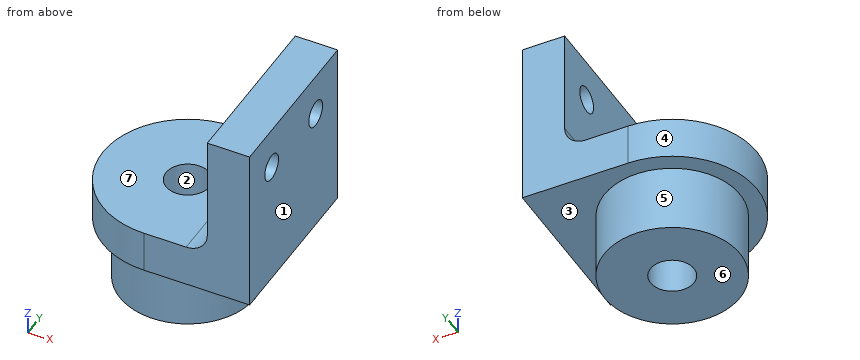
Autodesk Inventor part; units mm, degrees
ref_plane "YZ Plane" through (0, 0, 0) normal (1, 0, 0) x (0, 1, 0)
ref_plane "XZ Plane" through (0, 0, 0) normal (0, 1, 0) x (-1, 0, 0)
ref_plane "XY Plane" through (0, 0, 0) normal (0, 0, 1) x (1, 0, 0)
sketch "Sketch1" plane through (0, 0, 0) normal (0, 0, 1) x (1, 0, 0)
  circle A0 centre (0, 0) radius 10.16
  circle A1 centre (0, 0) radius 8.7376
  dimension "d0" = 20.32
  dimension "d6" = 17.4752
extrude "Extrusion1" add sketch "Sketch1" along normal blind 10.16 contours A0 | A1
sketch "Sketch2" plane through (0, 0, 10.16) normal (0, 0, 1) x (1, 0, 0)
  circle A0 centre (0, 0) radius 10.16
  circle A1 centre (0, 0) radius 12.7 construction
  line L0 (0, 12.7) -> (15.875, 12.7)
  line L1 (15.875, 12.7) -> (15.875, -12.7)
  line L2 (15.875, -12.7) -> (0, -12.7)
  arc A2 (0, 12.7) -> (0, -12.7) centre (0, 0) ccw
  point P0 (15.875, 0)
  dimension "d3" = 2.54
  dimension "d14" = 15.875
  dimension "d35" = 25.4
extrude "Extrusion2" add sketch "Sketch2" along normal blind 6.35 contours A0 | L0 L1 L2 A2
sketch "Sketch4" plane through (0, 0, 16.51) normal (0, 0, 1) x (1, 0, 0)
  arc A0 (0, 12.7) -> (0, -12.7) centre (0, 0) ccw
hole "Hole2" at (0, 0, 16.51) direction (0, 0, -1) diameter 6.5278 end through all
sketch "Sketch5" plane through (0, 0, 16.51) normal (0, 0, 1) x (1, 0, 0)
  line L0 (15.875, 12.7) -> (0, 12.7)
  line L1 (0, -12.7) -> (15.875, -12.7)
  line L2 (15.875, 12.7) -> (9.525, 12.7)
  line L3 (9.525, 12.7) -> (9.525, -12.7)
  line L4 (9.525, -12.7) -> (15.875, -12.7)
  line L5 (15.875, -12.7) -> (15.875, 12.7)
  point P0 (0, 0)
  dimension "d22" = 6.35
extrude "Extrusion3" add sketch "Sketch5" along normal blind 19.05
fillet "Fillet1" radius 3.175 1 edges at (9.525, 0, 16.51)
sketch "Sketch6" plane through (15.875, -12.7, 10.16) normal (1, 0, 0) x (0, 0, -1)
  line L0 (-19.05, 19.05) -> (-19.05, 6.35) construction
  line L1 (-25.4, 0) -> (-25.4, 25.4) construction
  line L2 (0, 25.4) -> (-25.4, 25.4) construction
  point P0 (10.16, 12.7)
  point P1 (-19.05, 12.7)
  point P2 (-25.4, 12.7)
  point P3 (-12.7, 25.4)
  dimension "d26" = 12.7
  dimension "d34" = 6.35
hole "Hole3" at (15.875, 6.35, 29.21) at (15.875, -6.35, 29.21) direction (-1, 0, 0) diameter 3.9624 end through all
properties part number "constant force Spring Holder" material "ABS Plastic"
Check sheet for the modelled part. Datum: model origin and axes. Units: mm. Face numbers are marked on the shaded views. A direction names the side the tool comes from. Round coordinates to 2 decimals unless told otherwise and drop trailing zeros. Loops run counter-clockwise (first coordinate to the right, second up) from the corner with the lowest first, then second, coordinate; pieces in that order, holes last.
1. Set-up check for the marked faces 5, 6 and 7: record each of +Z, -Z, +X, -X, +Y, -Y from which the full face is reachable in a straight line by a thin tool's end or side.
2. Gauge pin test, flat ends, axial feed: pin 1 Ø4.5 at (y, z) = (6.35, 29.21) entering from -X (3 decimals); pin 2 Ø3 at (x, y) = (-2.5, -0.5) entering from +Z; pin 3 Ø3 at (x, z) = (-4.5, 13.5) entering from +Y. Record the tip position at first contact, or that the pin passes through.
3. Sectioned sample at C-C on x = -2.5. Record the boundary of the cut face in (y, z).
4. Sectioned sample at B-B on y = 0. Record the boundary of the cut face in (x, z) (3 decimals).
5. Mould release check, pull along X, two halves, no side actions. Record for the marked faces 1, 2, 3 and 4: released by +X, released by -X, zero draft, split by the parting line, or undercut.
6. Sectioned sample at D-D on x = 4.25. Record the boundary of the cut face in (y, z).
7. Sectioned sample at A-A on z = 29.21. Record the boundary of the cut face in (x, y) (3 decimals), and give its area (3 significant figures).
8. Scan lines: probe 1 along Y at (x, z) = (14.75, 29.21); probe 2 along Y at (x, z) = (0, 5); probe 3 along Z at (x, y) = (14.25, -6.35). Record each from-to range of solid material in increasing order.
Recorded:
1. face 5: -Z
1. face 6: -Z, +X, -X, +Y, -Y
1. face 7: +Z, -X, +Y, -Y
2. pin 1: stops at x = 9.525
2. pin 2: stops at z = 16.51
2. pin 3: stops at y = 12.34
3. outline: (-12.45, 10.16) - (-9.85, 10.16) - (-9.85, 0) - (-2.1, 0) - (-2.1, 16.51) - (-12.45, 16.51) - close; (2.1, 0) - (9.85, 0) - (9.85, 10.16) - (12.45, 10.16) - (12.45, 16.51) - (2.1, 16.51) - close
4. outline: (-12.7, 10.16) - (-10.16, 10.16) - (-10.16, 0) - (-3.264, 0) - (-3.264, 16.51) - (-12.7, 16.51) - close; (3.264, 0) - (10.16, 0) - (10.16, 10.16) - (15.875, 10.16) - (15.875, 35.56) - (9.525, 35.56) - (9.525, 19.685) arc R3.175 cw to (6.35, 16.51) - (3.264, 16.51) - close
5. face 1: released by +X
5. face 2: undercut
5. face 3: zero draft
5. face 4: released by -X
6. outline: (-12.7, 10.16) - (-9.23, 10.16) - (-9.23, 0) - (9.23, 0) - (9.23, 10.16) - (12.7, 10.16) - (12.7, 16.51) - (-12.7, 16.51) - close
7. outline: (9.525, -12.7) - (15.875, -12.7) - (15.875, -8.331) - (9.525, -8.331) - close; (9.525, -4.369) - (15.875, -4.369) - (15.875, 4.369) - (9.525, 4.369) - close; (9.525, 8.331) - (15.875, 8.331) - (15.875, 12.7) - (9.525, 12.7) - close
7. area: 111 mm2
8. probe 1: y = -12.7 to -8.33, -4.37 to 4.37, 8.33 to 12.7
8. probe 2: y = -10.16 to -3.26, 3.26 to 10.16
8. probe 3: z = 10.16 to 27.23, 31.19 to 35.56
